Verification items for the finished model (mm, model axes). Face numbers are marked on the shaded views. Round coordinates to 2 decimals unless told otherwise and drop trailing zeros. Loops run counter-clockwise (first coordinate to the right, second up) from the corner with the lowest first, then second, coordinate; pieces in that order, holes last.
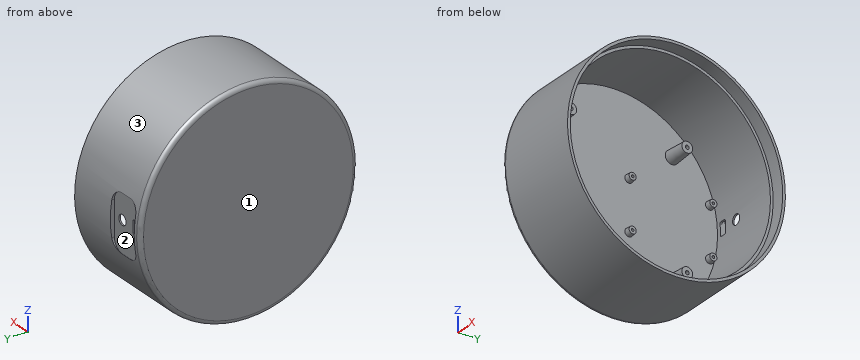
from build123d import *

# Parameters (mm, degrees)
SKETCH1_R           = 81
BOSS_EXTRUDE1_DEPTH = 2.5
SKETCH2_R           = 81
SKETCH2_R_2         = 77
BOSS_EXTRUDE2_DEPTH = 65.5
SKETCH4_R           = 5
BOSS_EXTRUDE3_DEPTH = 16
BOSS_EXTRUDE3_TAPER = 3.5
SKETCH6_R           = 1.4
CUT_EXTRUDE2_DEPTH  = 7
SKETCH7_R           = 79
CUT_EXTRUDE3_DEPTH  = 10
FILLET1_R           = 3
SKETCH8_R           = 3
BOSS_EXTRUDE4_DEPTH = 4
BOSS_EXTRUDE4_TAPER = 5
SKETCH9_R           = 1
CUT_EXTRUDE4_DEPTH  = 3
CUT_EXTRUDE5_DEPTH  = 3
CUT_EXTRUDE7_DEPTH  = 3
SKETCH15_R          = 3.75
CUT_EXTRUDE8_DEPTH  = 3


with BuildPart() as part:
    # Sketch1 → Boss-Extrude1 (new body)
    with BuildSketch(Plane(origin=(0, 0, 0), x_dir=(0, 0, -1), z_dir=(1, 0, 0))):
        Circle(SKETCH1_R)
    extrude(amount=BOSS_EXTRUDE1_DEPTH)

    # Sketch2 → Boss-Extrude2 (add)
    with BuildSketch(Plane(origin=(2.5, 0, 0), x_dir=(0, 0, -1), z_dir=(1, 0, 0))):
        Circle(SKETCH2_R)
        Circle(SKETCH2_R_2, mode=Mode.SUBTRACT)
    extrude(amount=BOSS_EXTRUDE2_DEPTH)

    # Sketch4 → Boss-Extrude3 (add)
    with BuildSketch(Plane(origin=(2.5, 0, 0), x_dir=(0, 0, -1), z_dir=(1, 0, 0))):
        with Locations((43.14, 43.135)):
            Circle(SKETCH4_R)
        with Locations((-43.14, 43.135)):
            Circle(SKETCH4_R)
        with Locations((43.14, -43.135)):
            Circle(SKETCH4_R)
        with Locations((-43.14, -43.135)):
            Circle(SKETCH4_R)
    extrude(amount=BOSS_EXTRUDE3_DEPTH, taper=BOSS_EXTRUDE3_TAPER)

    # Sketch6 → Cut-Extrude2 (cut)
    with BuildSketch(Plane(origin=(18.5, 0, 0), x_dir=(0, 0, -1), z_dir=(1, 0, 0))):
        with Locations((-43.14, 43.135)):
            Circle(SKETCH6_R)
        with Locations((43.14, 43.135)):
            Circle(SKETCH6_R)
        with Locations((-43.14, -43.135)):
            Circle(SKETCH6_R)
        with Locations((43.14, -43.135)):
            Circle(SKETCH6_R)
    extrude(amount=-CUT_EXTRUDE2_DEPTH, mode=Mode.SUBTRACT)

    # Sketch7 → Cut-Extrude3 (cut)
    with BuildSketch(Plane(origin=(68, 0, 0), x_dir=(0, 0, -1), z_dir=(1, 0, 0))):
        Circle(SKETCH7_R)
    extrude(amount=-CUT_EXTRUDE3_DEPTH, mode=Mode.SUBTRACT)

    # Fillet1
    fillet1_edges = [part.edges().sort_by_distance(p)[0] for p in [
        (0, 0, 81),
    ]]
    fillet(fillet1_edges, radius=FILLET1_R)

    # Sketch8 → Boss-Extrude4 (add)
    with BuildSketch(Plane(origin=(2.5, 0, 0), x_dir=(0, 0, -1), z_dir=(1, 0, 0))):
        with Locations((18.48, 71.045884469)):
            Circle(SKETCH8_R)
        with Locations((-18.48, 71.045884469)):
            Circle(SKETCH8_R)
        with Locations((18.48, 11.045884469)):
            Circle(SKETCH8_R)
        with Locations((-18.48, 11.045884469)):
            Circle(SKETCH8_R)
    extrude(amount=BOSS_EXTRUDE4_DEPTH, taper=BOSS_EXTRUDE4_TAPER)

    # Sketch9 → Cut-Extrude4 (cut)
    with BuildSketch(Plane(origin=(6.5, 0, 0), x_dir=(0, 0, -1), z_dir=(1, 0, 0))):
        with Locations((18.48, 71.045884469)):
            Circle(SKETCH9_R)
        with Locations((-18.48, 71.045884469)):
            Circle(SKETCH9_R)
        with Locations((-18.48, 11.045884469)):
            Circle(SKETCH9_R)
        with Locations((18.48, 11.045884469)):
            Circle(SKETCH9_R)
    extrude(amount=-CUT_EXTRUDE4_DEPTH, mode=Mode.SUBTRACT)

    # Sketch10 → Cut-Extrude5 (cut)
    with BuildSketch(Plane(origin=(0, 81, 0), x_dir=(1, 0, 0), z_dir=(0, 1, 0))):
        with BuildLine():
            Line((13.5, 21), (22.5, 21))
            ThreePointArc((22.5, 21), (28.156854249, 18.656854249), (30.5, 13))
            Line((30.5, 13), (30.5, -13))
            ThreePointArc((30.5, -13), (28.156854249, -18.656854249), (22.5, -21))
            Line((22.5, -21), (13.5, -21))
            ThreePointArc((13.5, -21), (7.843145751, -18.656854249), (5.5, -13))
            Line((5.5, -13), (5.5, 13))
            ThreePointArc((5.5, 13), (7.843145751, 18.656854249), (13.5, 21))
        make_face()
    extrude(amount=-CUT_EXTRUDE5_DEPTH, mode=Mode.SUBTRACT)

    # Sketch14 → Cut-Extrude7 (cut)
    with BuildSketch(Plane(origin=(0, 78, 0), x_dir=(1, 0, 0), z_dir=(0, 1, 0))):
        with BuildLine():
            Line((6.5, 2.5), (10, 2.5))
            ThreePointArc((10, 2.5), (10.707106781, 2.207106781), (11, 1.5))
            Line((11, 1.5), (11, -6.5))
            ThreePointArc((11, -6.5), (10.707106781, -7.207106781), (10, -7.5))
            Line((10, -7.5), (6.5, -7.5))
            ThreePointArc((6.5, -7.5), (5.792893219, -7.207106781), (5.5, -6.5))
            Line((5.5, -6.5), (5.5, 1.5))
            ThreePointArc((5.5, 1.5), (5.792893219, 2.207106781), (6.5, 2.5))
        make_face()
    extrude(amount=-CUT_EXTRUDE7_DEPTH, mode=Mode.SUBTRACT)

    # Sketch15 → Cut-Extrude8 (cut)
    with BuildSketch(Plane(origin=(0, 78, 0), x_dir=(1, 0, 0), z_dir=(0, 1, 0))):
        with Locations((22.046973968, -2.305883158)):
            Circle(SKETCH15_R)
    extrude(amount=-CUT_EXTRUDE8_DEPTH, mode=Mode.SUBTRACT)


solid = part.part
1. Section check B-B (x = 53). Enter the section's corners in (y, z), then the cut area to 3 significant figures.
2. Release check for a two-part mould opening along Z. For the marked faces 1, 2 and 3 record: released by +Z, released by -Z, zero draft, split by the parting line, or undercut.
3. Gauge pin test, flat ends, axial feed: P1, Ø4, axis at y = -41.5, z = 42, coming from the +X side; P2, Ø1.4, axis at y = 43, z = -43, coming from the +X side; P3, Ø12, axis at x = 8.5, z = -48.5, coming from the -Y side. Record the tip position at first contact, or that the pin passes through.
4. Section check A-A (y = 0). Enter the section's corners in (x, z), then the cut area to 3 significant figures.
5. Scan lines: L1, parallel to Z at x = 4, y = 45; L2, parallel to Y at x = 13, z = -43.14 (3 decimals); L3, parallel to Y at x = 51, z = -1. Record each from-to range of solid material in increasing order.
Taken from the geometry:
1. outline: circle Ø162 at (0, 0); hole circle Ø154 at (0, 0)
1. area: 1,990 mm2
2. face 1: zero draft
2. face 2: undercut
2. face 3: split by the parting line
3. P1: stops at x = 18.5
3. P2: stops at x = 11.5
3. P3: stops at y = -68.95
4. outline: (0, -78) arc R3 ccw to (3, -81) - (68, -81) - (68, -79) - (58, -79) - (58, -77) - (2.5, -77) - (2.5, 77) - (58, 77) - (58, 79) - (68, 79) - (68, 81) - (3, 81) arc R3 ccw to (0, 78) - close
4. area: 885 mm2
5. L1: z = -67.35 to -62.48, -47.68 to -38.6, 38.6 to 47.68, 62.48 to 67.35
5. L2: y = -68.556 to -63.78, -47.493 to -44.535, -41.735 to -38.777, 38.777 to 41.735, 44.535 to 47.493, 63.78 to 68.556
5. L3: y = -80.99 to -76.99, 76.99 to 80.99
